Verification items for the finished model (mm, model axes). Face numbers are marked on the shaded views. A direction names the side the tool comes from. Give positions to 0.01 mm unless a question says otherwise; leave off trailing zeros. Write each loop counter-clockwise with the first axis right and the second up, starting at its lowest first coordinate (ties: lowest second). Pieces come first, ordered by that corner, then holes.
from build123d import *

# Parameters (mm, degrees)
PAD_DEPTH       = 128
SKETCH001_W     = 8
SKETCH001_H     = 40
POCKET_DEPTH    = 20.001
SKETCH002_W     = 50
SKETCH002_H     = 14
PAD001_DEPTH    = 8
SKETCH003_R     = 8
POCKET001_DEPTH = 100.001
POCKET002_DEPTH = 71.001


with BuildPart() as part:
    # Sketch → Pad (new body)
    with BuildSketch(Plane.XZ):
        with BuildLine():
            Line((-50, 100), (-50, 20))
            Line((-50, 20), (-66, 20))
            Line((-66, 20), (-66, 0))
            Line((-66, 0), (-40, 0))
            Line((-40, 0), (-40, 40))
            ThreePointArc((40, 40), (0, 80), (-40, 40))
            Line((40, 0), (40, 40))
            Line((66, 0), (40, 0))
            Line((66, 20), (66, 0))
            Line((50, 20), (66, 20))
            Line((50, 20), (50, 100))
            Line((50, 100), (-50, 100))
        make_face()
    extrude(amount=PAD_DEPTH)

    # Sketch001 (on Face12 of Pad) → Pocket (cut, through all)
    with BuildSketch(Plane(origin=(0, 0, 20), x_dir=(-1, 0, 0), z_dir=(0, 0, 1))):
        with Locations((-62, 64)):
            Rectangle(SKETCH001_W, SKETCH001_H)
        with Locations((62, 64)):
            Rectangle(SKETCH001_W, SKETCH001_H)
    extrude(amount=-POCKET_DEPTH, mode=Mode.SUBTRACT)

    # Sketch002 (on Face1 of Pocket) → Pad001 (join)
    with BuildSketch(Plane(origin=(50, 0, 0), x_dir=(0, 0, 1), z_dir=(1, 0, 0))):
        with Locations((45, 64)):
            Rectangle(SKETCH002_W, SKETCH002_H)
    extrude(amount=PAD001_DEPTH)

    # Sketch003 (on Face3 of Pad001) → Pocket001 (cut, through all)
    with BuildSketch(Plane(origin=(0, 0, 100), x_dir=(-1, 0, 0), z_dir=(0, 0, 1))):
        with Locations((0, 64)):
            Circle(SKETCH003_R)
    extrude(amount=-POCKET001_DEPTH, mode=Mode.SUBTRACT)

    # Sketch004 (on Face6 of Pocket001) → Pocket002 (cut, through all)
    with BuildSketch(Plane.XZ.offset(71)):
        Polygon((58, 20), (58, 70), (50, 70), align=None)
    extrude(amount=-POCKET002_DEPTH, mode=Mode.SUBTRACT)

    # Mirrored: part across YZ


with BuildPart() as part_1:
    add(part.part)
    add(part.part.mirror(Plane.YZ))


solid = part_1.part
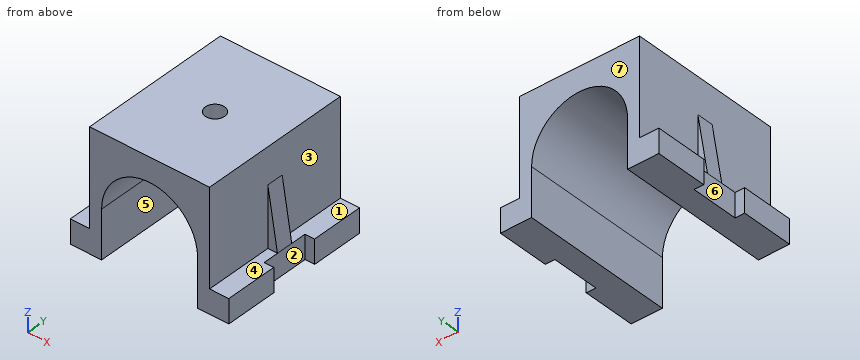
Item 1: Scan lines: line 1 along X through (y, z) = (-64, 87.5); line 2 along Y through (x, z) = (0, 91); line 3 along X through (y, z) = (-39, 31). Record each from-to range of solid material in increasing order.
Answer key:
line 1: x = -50 to -8, 8 to 50
line 2: y = -128 to -72, -56 to 0
line 3: x = -50 to -40, 40 to 50
Item 2: Set-up check for the marked faces 1, 2, 3 and 4: record each of +Z, -Z, +X, -X, +Y, -Y from which the full face is reachable in a straight line by a thin tool's end or side.
Answer key:
face 1: +Z, +X, +Y
face 2: +Z, -Z, +X
face 3: +Z, +X
face 4: +Z, +X, -Y
Item 3: Sectioned sample at C-C on z = 47. Record the cut outline in (x, y), then the cut area to 3 significant figures.
Answer key:
outline: (-53.68, -71) - (-50, -71) - (-50, -128) - (-39.38, -128) - (-39.38, 0) - (-50, 0) - (-50, -57) - (-53.68, -57) - close; (39.38, -128) - (50, -128) - (50, -71) - (53.68, -71) - (53.68, -57) - (50, -57) - (50, 0) - (39.38, 0) - close
area: 2,820 mm2
Item 4: Sectioned sample at B-B on x = 0. Record the cut outline in (y, z), then the cut area to 3 significant figures.
Answer key:
outline: (-128, 80) - (-72, 80) - (-72, 100) - (-128, 100) - close; (-56, 80) - (0, 80) - (0, 100) - (-56, 100) - close
area: 2,240 mm2
Item 5: Sectioned sample at A-A on y = -64. Record the cut outline in (x, z).
Answer key:
outline: (-58, 0) - (-40, 0) - (-40, 40) arc R40 cw to (-8, 79.19) - (-8, 100) - (-50, 100) - (-50, 70) - (-58, 20) - close; (8, 79.19) arc R40 cw to (40, 40) - (40, 0) - (58, 0) - (58, 20) - (50, 70) - (50, 100) - (8, 100) - close
Item 6: Sectioned sample at D-D on z = 88. Record the cut outline in (x, y), then the cut area to 3 significant figures.
Answer key:
outline: (-50, -128) - (50, -128) - (50, 0) - (-50, 0) - close; hole circle Ø16 at (0, -64)
area: 12,600 mm2
Item 7: Depth check by flat-ended pin: pin 1 (2.5 mm diameter, centred on x = 54.5, z = 40, fed in from +Y); pin 2 (2 mm diameter, centred on y = -110, z = 39, fed in from -X); pin 3 (8 mm diameter, centred on x = -11.5, y = -67, fed in from -Z). Enter the tip coordinate at first touch or a pass-through.
Answer key:
pin 1: stops at y = -57
pin 2: stops at x = -50
pin 3: stops at z = 76.87
Item 8: Release check for a two-part mould opening along Y. For the marked faces 5, 6 and 7 record: released by +Y, released by -Y, zero draft, split by the parting line, or undercut.
Answer key:
face 5: zero draft
face 6: undercut
face 7: released by +Y
